Autodesk Inventor part; units mm, degrees
ref_plane "YZ Plane" through (0, 0, 0) normal (1, 0, 0) x (0, 1, 0)
ref_plane "XZ Plane" through (0, 0, 0) normal (0, 1, 0) x (-1, 0, 0)
ref_plane "XY Plane" through (0, 0, 0) normal (0, 0, 1) x (1, 0, 0)
sketch "Sketch1" plane through (0, 0, 0) normal (0, 0, 1) x (1, 0, 0)
  circle A0 centre (0, 0) radius 78
extrude "Connector" add sketch "Sketch1" along normal blind 20
sketch "Sketch2" plane through (0, 0, 0) normal (0, 0, -1) x (-1, 0, 0)
  circle A0 centre (0, 0) radius 20
extrude "RotAxis" add sketch "Sketch2" along normal blind 624
sketch "Sketch3" plane through (0, 0, 20) normal (0, 0, 1) x (1, 0, 0)
  line L0 (78, 234) -> (-78, 234)
  line L1 (-78, 234) -> (-78, -156)
  line L2 (-78, -156) -> (78, -156)
  line L3 (78, -156) -> (78, 234)
  point P0 (0, 0)
extrude "TelescopeMount" add sketch "Sketch3" along normal blind 8
sketch "Sketch4" plane through (0, 0, -624) normal (0, 0, -1) x (-1, 0, 0)
  circle A0 centre (0, 0) radius 21
extrude "Cap" add sketch "Sketch4" along normal blind 8
properties part number "DecAxis"
Input: part model. Units: mm. Frame: model coordinates. A direction names the side the tool comes from. Give positions to 0.01 mm unless a question says otherwise; leave off trailing zeros. Order: outer loops, then holes, each group sorted by start corner. A loop starts at its lowest first (then second) coordinate and runs counter-clockwise, first axis right, second up. Notation, with made-up numbers: M -32.5,31 L -14.5,31 A22 cw -14.5,59 Z; hole C 2.25,77 d10. An arc over 180 degrees is marked long. Answer as a JSON object with one key per item and string values.
1. Cut plane B-B, the plane y = -45.5. Output: boundary loops of the cut face in (x, z), and give its area (3 significant figures).
Result sheet:
{"outline": "M -78,20 L -63.35,20 L -63.35,0 L 63.35,0 L 63.35,20 L 78,20 L 78,28 L -78,28 Z", "area": "3,780 mm²"}
2. Ray query, line 1 (Z direction, x = -30, y = 1); line 2 (Z direction, x = 54, y = 57.5); line 3 (X direction, y = -17.5, z = -33). Return the intervals inside material, ascending. Write a range as [from, to].
Result sheet:
{"line 1": "[0, 28]", "line 2": "[20, 28]", "line 3": "[-9.68, 9.68]"}
3. Pull-direction query (Z, two-part tool) for faces 1 (the flat face through (-1, 145, 20)), 2 (the flat face through (-1, 42, 28)), 3 (the flat face through (-19, -8, -624)), 4 (the cylindrical face through (4.336, 19.524, -307.632)); classes: +Z half, -Z half, draft (parallel to the pull), parting line (faces both ways), or undercut.
Result sheet:
{"face 1": "-Z half", "face 2": "+Z half", "face 3": "undercut", "face 4": "undercut"}
4. First-contact query: P1, Ø6, axis at x = -50.5, y = -81.5, coming from the -Z side; P2, Ø8, axis at y = -0.5, z = -533.5, coming from the +X side; P3, Ø12, axis at x = -8.5, z = -546, coming from the -Y side. Flat tips, straight axial feed; report the tip coordinate or a pass-through.
Result sheet:
{"P1": "z = 20", "P2": "x = 20", "P3": "y = -19.84"}
5. Cut plane C-C, the plane z = -88. Output: boundary loops of the cut face in (x, y).
Result sheet:
{"outline": "C 0,0 d40"}
6. Cut plane A-A, the plane x = 0. Output: boundary loops of the cut face in (y, z).
Result sheet:
{"outline": "M -156,20 L -78,20 L -78,0 L -20,0 L -20,-624 L -21,-624 L -21,-632 L 21,-632 L 21,-624 L 20,-624 L 20,0 L 78,0 L 78,20 L 234,20 L 234,28 L -156,28 Z"}
7. Cut plane D-D, the plane x = 53.5. Output: boundary loops of the cut face in (y, z).
Result sheet:
{"outline": "M -156,20 L -56.76,20 L -56.76,0 L 56.76,0 L 56.76,20 L 234,20 L 234,28 L -156,28 Z"}
8. Reachability of faces 5 (the flat face through (0, 0, -632)), 6 (the cylindrical face through (-20.03, -6.31, -627.94)), 7 (the flat face through (-1, -112, 20)) from +Z, -Z, +X, -X, +Y, -Y: full face, straight path, thin tool, end or side. Return the list, or none.
Result sheet:
{"face 5": "-Z, +X, -X, +Y, -Y", "face 6": "-Z", "face 7": "-Z, -Y"}
